```python
from build123d import *

# Parameters (mm, degrees)
BOSS_EXTRUDE1_DEPTH = 3.1
FILLET1_R           = 2.5
FILLET2_R           = 1.1
SKETCH2_R           = 4.304443881
SKETCH2_R_2         = 7.925342076
SKETCH2_W           = 29.557408324
SKETCH2_H           = 28.485114527
CUT_EXTRUDE1_DEPTH  = 4
FILLET3_R           = 0.7
FILLET4_R           = 1.1
FILLET5_R           = 2.9
FILLET6_R           = 20
FILLET7_R           = 5
FILLET8_R           = 1.8
SKETCH4_R           = 2.6
CUT_EXTRUDE2_DEPTH  = 130.682927753
FILLET9_R           = 0.6


with BuildPart() as part:
    # Sketch1 → Boss-Extrude1 (new body)
    with BuildSketch(Plane(origin=(0, 0, 0), x_dir=(0, 0, -1), z_dir=(1, 0, 0))):
        with BuildLine():
            Line((0, 0), (0, -3.1))
            Line((0, -3.1), (3, -3.1))
            Line((3, -3.1), (3, -8.1))
            Line((3, -8.1), (-25, -8.1))
            Line((-25, -8.1), (-25, 0))
            Line((-25, 0), (-65, 0))
            Line((-65, 0), (-65, -3.1))
            Line((-65, -3.1), (-62, -3.1))
            Line((-62, -3.1), (-62, -8.1))
            Line((-62, -8.1), (-78.979671767, -8.1))
            Line((-78.979671767, -8.1), (-78.979671767, 0))
            Line((-78.979671767, 0), (-82.880201339, 0))
            Line((-82.880201339, 0), (-117.70382886, 46.590063892))
            Line((-117.70382886, 46.590063892), (-104.111751507, 56.5))
            Line((-104.111751507, 56.5), (-96.111751507, 56.5))
            ThreePointArc((-96.111751507, 56.5), (-85.755593918, 40), (-75.39943633, 56.5))
            Line((-75.39943633, 56.5), (-66.111751507, 56.5))
            ThreePointArc((-66.111751507, 56.5), (-55.755593918, 40), (-45.39943633, 56.5))
            Line((-45.39943633, 56.5), (-35.299167427, 56.5))
            Line((-35.299167427, 56.5), (4.130048311, 3.748181445))
            Line((4.130048311, 3.748181445), (4.130048311, 0))
            Line((4.130048311, 0), (0, 0))
        make_face()
    extrude(amount=BOSS_EXTRUDE1_DEPTH)

    # Fillet1
    fillet1_edges = [part.edges().sort_by_distance(p)[0] for p in [
        (1.55, 0, 82.880201339),
        (1.55, 46.590063892, 117.70382886),
        (1.55, 56.5, 104.111751507),
        (1.55, 56.5, 96.111751507),
        (1.55, 56.5, 75.39943633),
        (1.55, 56.5, 66.111751507),
        (1.55, 56.5, 45.39943633),
        (1.55, 56.5, 35.299167427),
        (1.55, 3.748181445, -4.130048311),
    ]]
    fillet(fillet1_edges, radius=FILLET1_R)

    # Fillet2
    fillet2_edges = [part.edges().sort_by_distance(p)[0] for p in [
        (1.55, 0, -4.130048311),
    ]]
    fillet(fillet2_edges, radius=FILLET2_R)

    # Sketch2 → Cut-Extrude1 (cut)
    with BuildSketch(Plane(origin=(3.1, 0, 0), x_dir=(0, 0, -1), z_dir=(1, 0, 0))):
        with Locations((-97.418386441, 32.55612307)):
            Circle(SKETCH2_R)
        with Locations((-77.029808816, 15.272951492)):
            Circle(SKETCH2_R_2)
        with Locations((-82.418386441, 32.55612307)):
            Circle(SKETCH2_R)
        with Locations((-67.418386441, 32.55612307)):
            Circle(SKETCH2_R)
        with BuildLine():
            Line((-78.979671767, -2.567225462), (-75.079945866, -2.567225462))
            ThreePointArc((-75.079945866, -2.567225462), (-73.597171327, -4.05), (-75.079945866, -5.532774538))
            Line((-75.079945866, -5.532774538), (-78.979671767, -5.532774538))
            ThreePointArc((-78.979671767, -5.532774538), (-80.462446305, -4.05), (-78.979671767, -2.567225462))
        make_face()
        with Locations((-46.829052789, 14.242557264)):
            Rectangle(SKETCH2_W, SKETCH2_H)
    extrude(amount=-CUT_EXTRUDE1_DEPTH, mode=Mode.SUBTRACT)

    # Fillet3
    fillet3_edges = [part.edges().sort_by_distance(p)[0] for p in [
        (1.55, -2.567225462, 78.979671767),
        (1.55, -5.532774538, 78.979671767),
    ]]
    fillet(fillet3_edges, radius=FILLET3_R)

    # Fillet4
    fillet4_edges = [part.edges().sort_by_distance(p)[0] for p in [
        (1.55, -3.1, 0),
        (1.55, -3.1, -3),
        (1.55, -3.1, 65),
        (1.55, -3.1, 62),
    ]]
    fillet(fillet4_edges, radius=FILLET4_R)

    # Fillet5
    # the kernel refuses this fillet: 2.9 mm, written as the material it takes off along each edge
    with BuildSketch(Plane(origin=(-7.25, -8.1, -3), x_dir=(0, 0, 1), z_dir=(1, 0, 0)), Plane(origin=(-7.25, -8.1, 25), x_dir=(0, 1, 0), z_dir=(1, 0, 0))) as fillet5_piece_1:
        with BuildLine():
            CenterArc((FILLET5_R, -FILLET5_R), FILLET5_R, 90, 90)
            Line((0, -FILLET5_R), (0, 0))
            Line((0, 0), (FILLET5_R, 0))
        make_face()
    extrude(amount=17.6, mode=Mode.SUBTRACT)
    with BuildSketch(Plane(origin=(-7.25, -8.1, 62), x_dir=(0, 1, 0), z_dir=(1, 0, 0))) as fillet5_piece_2:
        with BuildLine():
            CenterArc((FILLET5_R, FILLET5_R), FILLET5_R, 180, 90)
            Line((0, FILLET5_R), (0, 0))
            Line((0, 0), (FILLET5_R, 0))
        make_face()
    extrude(amount=17.6, mode=Mode.SUBTRACT)
    with BuildSketch(Plane(origin=(-6.774666391, -8.1, 78.979671767), x_dir=(0, 0, -1), z_dir=(1, 0, 0))) as fillet5_piece_3:
        with BuildLine():
            CenterArc((2.709866556, 2.9), FILLET5_R, 200.862663323, 69.137336677)
            Line((0, 1.867225462), (0, 0))
            Line((0, 0), (2.709866556, 0))
        make_face()
    extrude(amount=16.649332781, mode=Mode.SUBTRACT)

    # Fillet6
    fillet6_edges = [part.edges().sort_by_distance(p)[0] for p in [
        (1.55, 28.485114527, 32.050348627),
    ]]
    fillet(fillet6_edges, radius=FILLET6_R)

    # Fillet7
    fillet7_edges = [part.edges().sort_by_distance(p)[0] for p in [
        (1.55, 28.485114527, 61.607756951),
    ]]
    fillet(fillet7_edges, radius=FILLET7_R)

    # Fillet8
    fillet8_edges = [part.edges().sort_by_distance(p)[0] for p in [
        (1.55, 0, 61.607756951),
        (1.55, 0, 32.050348627),
    ]]
    fillet(fillet8_edges, radius=FILLET8_R)

    # Sketch4 → Cut-Extrude2 (cut, through all)
    with BuildSketch(Plane(origin=(3.1, 0, 0), x_dir=(0, 0, -1), z_dir=(1, 0, 0))):
        with Locations((-28.303725911, 35.631276326)):
            Circle(SKETCH4_R)
        with Locations((-21.045298439, 25.920323627)):
            Circle(SKETCH4_R)
        with Locations((-13.786870968, 16.209370928)):
            Circle(SKETCH4_R)
        with Locations((-6.528443496, 6.498418229)):
            Circle(SKETCH4_R)
        with BuildLine():
            Line((-35.562153383, 47.942229025), (-28.90268277, 47.942229025))
            Line((-28.90268277, 47.942229025), (-25.015955687, 42.742229025))
            Line((-25.015955687, 42.742229025), (-35.562153383, 42.742229025))
            ThreePointArc((-35.562153383, 42.742229025), (-38.162153383, 45.342229025), (-35.562153383, 47.942229025))
        make_face()
        with BuildLine():
            Line((-112.340464073, 39.414490126), (-108.529774826, 42.262780338))
            ThreePointArc((-108.529774826, 42.262780338), (-105.030597304, 41.757056436), (-105.536321205, 38.257878913))
            Line((-105.536321205, 38.257878913), (-109.347010452, 35.409588702))
            ThreePointArc((-109.347010452, 35.409588702), (-112.846187975, 35.915312603), (-112.340464073, 39.414490126))
        make_face()
    extrude(amount=-CUT_EXTRUDE2_DEPTH, mode=Mode.SUBTRACT)

    # Fillet9
    fillet9_edges = [part.edges().sort_by_distance(p)[0] for p in [
        (1.55, 47.942229025, 28.90268277),
        (1.55, 42.742229025, 25.015955687),
        (1.55, 35.409588702, 109.347010452),
        (1.55, 39.414490126, 112.340464073),
    ]]
    fillet(fillet9_edges, radius=FILLET9_R)


solid = part.part
```
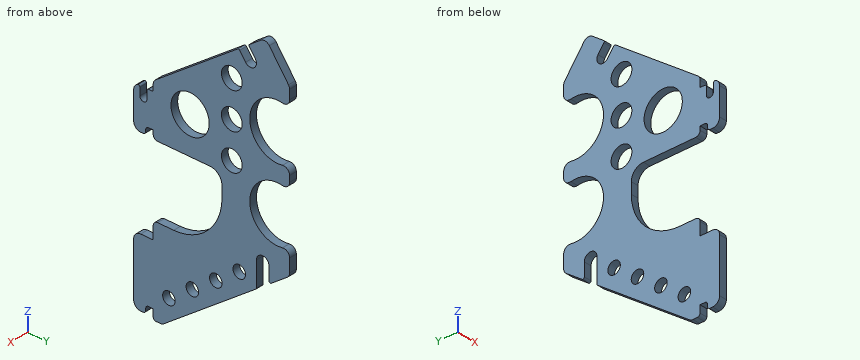
Could you check a few things on this model? Use its own coordinates, in mm. Round coordinates to 2 decimals unless told otherwise and drop trailing zeros. Order: outer loops, then holes, each group sorted by start corner. A loop starts at its lowest first (then second) coordinate and runs counter-clockwise, first axis right, second up. Notation, with made-up numbers: (38, -39.75) -> (74, -39.75) arc R11 ccw to (74, -22.75) -> close; hole circle Ø5 at (20.5, 32). An arc over 180 degrees is marked (long way). One line per question, with ' | ' between items.
Q1. I'm going to push flat-ended pins straight in: pin 1 (0.9 mm diameter, centred on x = 2, z = -2, fed in from -Y); pin 2 (1.6 mm diameter, centred on x = 2, z = 76.5, fed in from +Y); pin 3 (0.6 mm diameter, centred on x = 1.5, y = -1.5, fed in from -Z). Where does each tip first touch, or does it pass through?
Computed values:
pin 1: y = -7.71 | pin 2: y = 45.92 | pin 3: z = 0
Q2. If we section it at C-C on z = 91: Write out the boundary of the cut face in (x, y), plus the area to 3 significant figures.
Computed values:
outline: (0, 10.86) -> (3.1, 10.86) -> (3.1, 41.27) -> (0, 41.27) -> close | area: 94.2 mm²
Q3. If we section it at D-D on x = 0.8: Give the number of separate pieces and of enclosed holes in the cut face, plus the area to 3 significant figures.
Computed values:
separate pieces: 1 | enclosed holes: 8 | area: 3,340 mm²
Q4. If I drill on line 1 (Z direction, x = 1.4, y = 7); line 2 (Z direction, x = 2.45, y = 51.5); line 3 (Z direction, x = 0.45, y = 42), over which ranges is the centre line in solid material (lowest first)? Write a range as from..to.
Computed values:
line 1: -1.7..3.98, 9.08..32.05, 61.61..88.11 | line 2: 31.56..44.26, 67.26..74.26, 97.26..110.97 | line 3: 24.46..49.27, 62.24..79.27, 92.24..105.24, 108.88..114.27
Q5. If we section it at A-A on y = 51.5: Write out the boundary of the cut face in (x, z), plus the area to 3 significant figures.
Computed values:
outline: (0, 31.56) -> (3.1, 31.56) -> (3.1, 44.26) -> (0, 44.26) -> close; (0, 67.26) -> (3.1, 67.26) -> (3.1, 74.26) -> (0, 74.26) -> close; (0, 97.26) -> (3.1, 97.26) -> (3.1, 110.97) -> (0, 110.97) -> close | area: 104 mm²
Q6. If we section it at B-B on z = 27: Write out the boundary of the cut face in (x, y).
Computed values:
outline: (0, 0) -> (3.1, 0) -> (3.1, 33.38) -> (0, 33.38) -> close; (0, 37.88) -> (3.1, 37.88) -> (3.1, 42.74) -> (0, 42.74) -> close
